For this review, take the finished solid that the model builds, in its own axes (mm). Round coordinates to 2 decimals unless told otherwise and drop trailing zeros. Loops run counter-clockwise (first coordinate to the right, second up) from the corner with the lowest first, then second, coordinate; pieces in that order, holes last. Notation, with made-up numbers: M 24.5,61 L 76.5,61 A16 cw 76.5,66 Z; hole C -33,-21.75 d10. An arc over 180 degrees is marked long. One line per question, with ' | ' between items. Start each with the question number.
1) We need section C-C (x = 27.5). Give the boundary of the cut face in (y, z), and give its area (3 significant figures).
2) We need section B-B (z = 1.4). Give the boundary of the cut face in (x, y).
3) We need section D-D (y = 12.5). Give the boundary of the cut face in (x, z).
4) We need section A-A (y = 0). Give the boundary of the cut face in (x, z), and give its area (4 significant figures).
5) For probe 1 along Y at (x, z) = (27.5, 2.05); probe 2 along X at (y, z) = (21, 2.45); probe 3 along X at (y, z) = (12, 2.5), list the stretches that pass through material, from the lowest coordinate up. Write a range as from..to.
```python
from build123d import *

# Parameters (mm, degrees)
SKETCH_W            = 70
SKETCH_H            = 55
PAD_DEPTH           = 3
SKETCH001_R         = 2.25
HOLE_DEPTH          = 25
HOLE001_D           = 4.5
HOLE001_DEPTH       = 25
HOLE001_CSINK_D     = 8.5
HOLE001_CSINK_ANGLE = 90
SKETCH003_R         = 4.25
HOLE002_DEPTH       = 25


with BuildPart() as part:
    # Sketch → Pad (new body)
    with BuildSketch(Plane.XY):
        Rectangle(SKETCH_W, SKETCH_H)
    extrude(amount=PAD_DEPTH)

    # Sketch001 (on Face6 of Pad) → Hole (cut)
    with BuildSketch(Plane.XY.offset(3)):
        with Locations((-27.5, 13.5)):
            Circle(SKETCH001_R)
        with Locations((-27.5, -13.5)):
            Circle(SKETCH001_R)
        with Locations((27.5, 13.5)):
            Circle(SKETCH001_R)
        with Locations((27.5, -13.5)):
            Circle(SKETCH001_R)
    extrude(amount=-HOLE_DEPTH, mode=Mode.SUBTRACT)

    # Hole001
    with Locations(Plane(origin=(0, 0, 0), x_dir=(1, 0, 0), z_dir=(0, 0, -1))):
        with Locations((0, 21), (0, -21)):
            CounterSinkHole(HOLE001_D / 2, HOLE001_CSINK_D / 2, depth=HOLE001_DEPTH, counter_sink_angle=HOLE001_CSINK_ANGLE)

    # Sketch003 (on Face5 of Hole001) → Hole002 (cut)
    with BuildSketch(Plane.XY.offset(3)):
        Circle(SKETCH003_R)
    extrude(amount=-HOLE002_DEPTH, mode=Mode.SUBTRACT)


solid = part.part
```
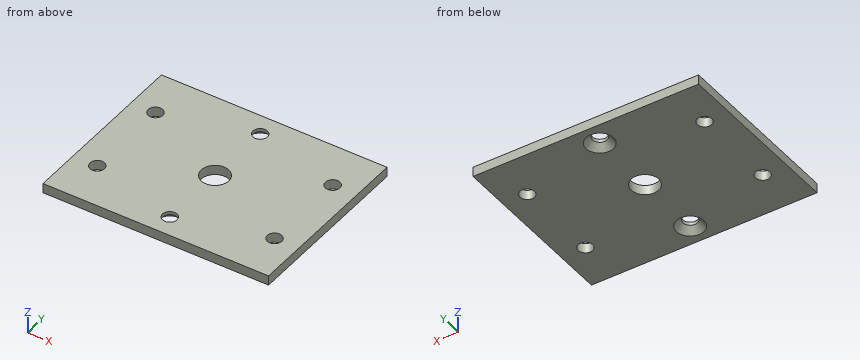
Answers below:
1) outline: M -27.5,0 L -15.75,0 L -15.75,3 L -27.5,3 Z; M -11.25,0 L 11.25,0 L 11.25,3 L -11.25,3 Z; M 15.75,0 L 27.5,0 L 27.5,3 L 15.75,3 Z | area: 138 mm^2
2) outline: M -35,-27.5 L 35,-27.5 L 35,27.5 L -35,27.5 Z; hole C -27.5,-13.5 d4.5; hole C -27.5,13.5 d4.5; hole C 0,0 d8.5; hole C 0,-21 d5.7; hole C 0,21 d5.7; hole C 27.5,-13.5 d4.5; hole C 27.5,13.5 d4.5
3) outline: M -35,0 L -29.52,0 L -29.52,3 L -35,3 Z; M -25.48,0 L 25.48,0 L 25.48,3 L -25.48,3 Z; M 29.52,0 L 35,0 L 35,3 L 29.52,3 Z
4) outline: M -35,0 L -4.25,0 L -4.25,3 L -35,3 Z; M 4.25,0 L 35,0 L 35,3 L 4.25,3 Z | area: 184.5 mm^2
5) probe 1: -27.5..-15.75, -11.25..11.25, 15.75..27.5 | probe 2: -35..-2.25, 2.25..35 | probe 3: -35..-29.18, -25.82..25.82, 29.18..35
